Autodesk Inventor part; units mm, degrees
ref_plane "YZ Plane" through (0, 0, 0) normal (1, 0, 0) x (0, 1, 0)
ref_plane "XZ Plane" through (0, 0, 0) normal (0, 1, 0) x (-1, 0, 0)
ref_plane "XY Plane" through (0, 0, 0) normal (0, 0, 1) x (1, 0, 0)
sketch "Sketch1" plane through (0, 0, 0) normal (0, 1, 0) x (-1, 0, 0)
  line L0 (36.9116, 5.5131) -> (-20.2384, 5.5131)
  line L1 (-20.2384, 5.5131) -> (-20.2384, -32.5869)
  line L2 (-20.2384, -32.5869) -> (36.9116, -32.5869)
  line L3 (36.9116, -32.5869) -> (36.9116, 5.5131)
  point P0 (0, 0)
  dimension "d0" = 57.15
  dimension "d1" = 38.1
extrude "Extrusion1" add sketch "Sketch1" along normal blind 31.75
sketch "Sketch2" plane through (0, 31.75, 0) normal (0, 1, 0) x (1, 0, 0)
  line L0 (-36.9116, -5.5131) -> (20.2384, -5.5131)
  line L1 (20.2384, -5.5131) -> (1.1884, -5.5131)
  line L2 (1.1884, -5.5131) -> (1.1884, 13.5369)
  line L3 (1.1884, 13.5369) -> (20.2384, 13.5369)
  line L4 (20.2384, 13.5369) -> (20.2384, -5.5131)
  line L5 (20.2384, -5.5131) -> (20.2384, 32.5869)
  line L6 (20.2384, 32.5869) -> (1.1884, 32.5869)
  line L7 (1.1884, 32.5869) -> (1.1884, 13.5369)
  line L8 (1.1884, 13.5369) -> (20.2384, 13.5369)
  line L9 (20.2384, 13.5369) -> (20.2384, 32.5869)
  point P0 (0, 0)
  dimension "d4" = 19.05
  dimension "d5" = 19.05
  dimension "d6" = 19.05
  dimension "d7" = 19.05
sketch "Sketch3" plane through (0, 31.75, 0) normal (0, 1, 0) x (1, 0, 0)
  line L0 (20.2384, -5.5131) -> (20.2384, 32.5869)
  circle A0 centre (20.2384, 13.5369) radius 12.7
  point P0 (0, 0)
  dimension "d8" = 25.4
extrude "Extrusion2" cut sketch "Sketch3" against normal blind 31.75
sketch "Sketch5" plane through (-36.9116, 0, -32.5869) normal (-1, 0, 0) x (0, 0, 1)
  line L0 (0, 0) -> (38.1, 0)
  line L1 (38.1, 0) -> (31.75, 0)
  line L2 (31.75, 0) -> (31.75, 6.35)
  line L3 (31.75, 6.35) -> (38.1, 6.35)
  line L4 (38.1, 6.35) -> (38.1, 0)
  line L5 (38.1, 0) -> (38.1, 31.75)
  circle A0 centre (38.1, 31.75) radius 25.4
  point P0 (32.5869, 0)
  dimension "d13" = 6.35
  dimension "d14" = 6.35
  dimension "d15" = 50.8
extrude "Extrusion3" cut sketch "Sketch5" against normal blind 25.4 contours A0
sketch "Sketch6" plane through (-36.9116, 0, 5.5131) normal (0, 0, 1) x (1, 0, 0)
  line L0 (25.4, 31.75) -> (57.15, 31.75)
  circle A0 centre (38.1, 19.05) radius 3.175
  point P0 (36.9116, 0)
  dimension "d20" = 6.35
extrude "Extrusion4" cut sketch "Sketch6" against normal blind 50.8
The listing builds one solid part. Answer for the finished solid, in the listing's coordinates (mm). A direction names the side the tool comes from. Round coordinates to 2 decimals unless told otherwise and drop trailing zeros. Write each loop counter-clockwise with the first axis right and the second up, starting at its lowest first coordinate (ties: lowest second). Pieces come first, ordered by that corner, then holes. Notation, with made-up numbers: (-36, 30.25) - (-10, 30.25) arc R14 ccw to (-10, 43.25) - close; hole circle Ø8 at (-30.5, 23.25). An arc over 180 degrees is marked (long way). Use a Markdown table: item, result. Add a question column.
1. The part is cut by section B-B (z = -8.5). Write down the section's boundary in (x, y) (3 decimals).
2. The part is cut by section A-A (x = -0.5). Write down the section's boundary in (y, z), and give its area (3 significant figures).
3. Flat-ended cylindrical pins translate along their axes: P1, Ø3, axis at x = -26, z = -24, coming from the -Y side; P2, Ø6, axis at y = 11, z = -5, coming from the +X side; P3, Ø4, axis at x = 1.19, y = 19.05, coming from the +Z side. Find the tip coordinate at first contact, or state that the pin passes through.
4. The part is cut by section D-D (x = -19.5). Write down the section's boundary in (y, z), and give its area (3 significant figures).
5. For a pull along X with two mould halves and no side action, classify faces 1 (the face through (-2, 31.75, -18)), 2 (the face through (7.54, 16.1, -13.82)), 3 (the face through (0.5, 15.95, -13.27)) as +X half, -X half, draft (parallel to the pull), parting line (faces both ways), or undercut.
6. The part is cut by section C-C (y = 19.05). Write down the section's boundary in (x, z), and give its area (3 significant figures).
7. Consider line 1 (Y direction, x = 1.5, z = 0); line 2 (X direction, y = 21, z = -3.5); line 3 (Y direction, x = 3.5, z = -27). Determine where each line is inside the solid, lowest interval first.
8. A tool of negligible diameter and unlimited length cuts with its end or side. For faces 4 (the face through (-11.512, 22, -5)), 5 (the face through (-36.912, 12, -18)), from which of +Z, -Z, +X, -X, +Y, -Y can it reach the whole face along a straight path? Write none if from no direction.
Reported:
| question | item | result |
|---|---|---|
| 1 | outline | (-36.912, 0) - (8.58, 0) - (8.58, 31.75) - (-11.512, 31.75) - (-11.512, 10.565) - (-36.912, 10.565) - close; hole circle Ø6.35 at (1.188, 19.05) |
| 2 | outline | (0, -32.59) - (16.36, -32.59) - (16.36, 5.51) - (0, 5.51) - close; (21.74, -32.59) - (31.75, -32.59) - (31.75, 5.51) - (21.74, 5.51) - close |
| 2 | area | 1,000 mm^2 |
| 3 | P1 | y = 0 |
| 3 | P2 | x = 14.93 |
| 3 | P3 | through |
| 4 | outline | (0, -32.59) - (31.75, -32.59) - (31.75, -19.89) arc R25.4 cw to (6.35, 5.51) - (0, 5.51) - close |
| 4 | area | 703 mm^2 |
| 5 | face 1 | draft |
| 5 | face 2 | +X half |
| 5 | face 3 | undercut |
| 6 | outline | (-36.91, -32.59) - (-1.99, -32.59) - (-1.99, 5.51) - (-11.51, 5.51) - (-11.51, -16.48) - (-36.91, -16.48) - close; (4.36, -32.59) - (20.24, -32.59) - (20.24, -26.24) arc R12.7 cw to (20.24, -0.84) - (20.24, 5.51) - (4.36, 5.51) - close |
| 6 | area | 1,120 mm^2 |
| 7 | line 1 | 0 to 15.89, 22.21 to 31.75 |
| 7 | line 2 | -11.51 to -1.32, 3.69 to 12.46 |
| 7 | line 3 | 0 to 16.87, 21.23 to 31.75 |
| 8 | face 4 | +Z, -X, +Y |
| 8 | face 5 | +Z, -Z, -X, +Y, -Y |
